Geometry: final body of the model. Coordinates: model frame, mm. Face numbers are marked on the shaded views. A direction names the side the tool comes from. Coordinates: 2 decimals unless noted, no trailing zeros. Order: outer loops, then holes, each group sorted by start corner. A loop starts at its lowest first (then second) coordinate and runs counter-clockwise, first axis right, second up. Notation, with made-up numbers: (28.5, 61.25) -> (60.5, 61.25) arc R27 cw to (60.5, 96.25) -> close; hole circle Ø7 at (8.25, -17.5). An arc over 180 degrees is marked (long way). Use CSV: the item, a comma, the result in double quotes. Start each with the question number.
Autodesk Inventor part; units mm, degrees
ref_plane "Work Plane1" through (0, 41.6, 0) normal (0, 1, 0) x (1, 0, 0)
ref_plane "Work Plane2" through (0, 50.6, 0) normal (0, 1, 0) x (1, 0, 0)
ref_plane "YZ Plane" through (0, 0, 0) normal (1, 0, 0) x (0, 1, 0)
sketch "Sketch1" plane through (0, 0, 0) normal (0, 1, 0) x (-1, 0, 0)
  circle A0 centre (0, 0) radius 13.75
  dimension "d0" = 27.5
extrude "Extrusion1" add sketch "Sketch1" along normal blind 46.6
sketch "Sketch2" plane through (0, 46.6, 0) normal (0, 1, 0) x (1, 0, 0)
  circle A0 centre (0, 0) radius 13.75
  circle A1 centre (0, 0) radius 5
  dimension "d3" = 10
extrude "Extrusion2" add sketch "Sketch2" along normal blind 3 contours A1
sketch "Sketch3" plane through (0, 46.6, 0) normal (0, 1, 0) x (1, 0, 0)
  circle A0 centre (0, 0) radius 5
  circle A1 centre (0, 0) radius 5
  circle A2 centre (0, 0) radius 13.75
  circle A3 centre (0, 0) radius 13.75
  line L0 (-13.75, 0) -> (13.75, 0)
  point P0 (-8, 0)
  point P1 (8, 0)
  dimension "d6" = 16
  dimension "d7" = 5.75
  dimension "d8" = 5.75
hole "Hole1" at (-8, 46.6, 0) at (8, 46.6, 0) direction (0, -1, 0) diameter 2.459 depth 3
ref_plane "Work Plane1" through (0, 41.6, 0) normal (0, 1, 0) x (1, 0, 0)
sketch "Sketch4" plane through (0, 41.6, 0) normal (0, 1, 0) x (1, 0, 0)
  circle A0 centre (0, 0) radius 15
  dimension "d17" = 30
extrude "Extrusion3" add sketch "Sketch4" against normal blind 27.7
sketch "Sketch5" plane through (0, 0, 0) normal (0, -1, 0) x (1, 0, 0)
  circle A0 centre (0, 0) radius 5
  dimension "d20" = 10
extrude "Extrusion4" add sketch "Sketch5" along normal blind 2.7
sketch "Sketch6" plane through (0, 0, 0) normal (0, -1, 0) x (1, 0, 0)
  circle A0 centre (0, 0) radius 5
  circle A1 centre (0, 0) radius 5
  circle A2 centre (0, 0) radius 13.75
  circle A3 centre (0, 0) radius 13.75
  line L0 (13.75, 0) -> (-13.75, 0)
  line L1 (-11.25, 1.35) -> (-11.75, 1.35)
  line L2 (-11.75, 1.35) -> (-11.75, -1.35)
  line L3 (-11.75, -1.35) -> (-11.25, -1.35)
  line L4 (-11.25, -1.35) -> (-11.25, 1.35)
  line L5 (11.25, 1.35) -> (10.75, 1.35)
  line L6 (10.75, 1.35) -> (10.75, -1.35)
  line L7 (10.75, -1.35) -> (11.25, -1.35)
  line L8 (11.25, -1.35) -> (11.25, 1.35)
  dimension "d23" = 22
  dimension "d24" = 0.5
  dimension "d25" = 0.5
  dimension "d26" = 11.25
  dimension "d27" = 11.25
  dimension "d28" = 2.7
  dimension "d29" = 2.7
  dimension "d30" = 1.35
  dimension "d31" = 1.35
extrude "Extrusion5" add sketch "Sketch6" along normal up to surface (2.7 mm away) contours L6 L5 L8 L0 | L0 L8 L7 L6 | L4 L3 L2 L0 | L0 L2 L1 L4
sketch "Sketch7" plane through (0, 49.6, 0) normal (0, 1, 0) x (1, 0, 0)
  circle A0 centre (0, 0) radius 1.15
  dimension "d34" = 2.3
extrude "Extrusion6" add sketch "Sketch7" along normal blind 9.5
ref_plane "Work Plane2" through (0, 50.6, 0) normal (0, 1, 0) x (1, 0, 0)
sketch "Sketch10" plane through (0, 0, 0) normal (1, 0, 0) x (0, 1, 0)
  line L0 (0, -13.75) -> (0, 13.75)
  line L1 (13.9, 13.75) -> (13.9, -13.75)
  line L2 (8.5, 3.8) -> (13.9, 3.8)
  line L3 (13.9, 3.8) -> (13.9, -3.8)
  line L4 (13.9, -3.8) -> (8.5, -3.8)
  line L5 (8.5, -3.8) -> (8.5, 3.8)
  circle A0 centre (11.2, 3.8) radius 2.7
  circle A1 centre (11.2, -3.8) radius 2.7
  line L6 (0, 0) -> (13.9, 0)
  line L7 (13.9, 13.75) -> (13.9, -13.75)
  line L8 (0, -13.75) -> (13.9, -13.75)
  point P0 (11.2, -6.5)
  point P1 (11.2, 6.5)
  dimension "d57" = 8.5
  dimension "d59" = 0
  dimension "d60" = 5.4
  dimension "d61" = 13.9
  dimension "d65" = 3.8
  dimension "d66" = 3.8
  dimension "d80" = 5.4
  dimension "d81" = 5.4
  dimension "d82" = 2.7
  dimension "d83" = 2.7
  dimension "d84" = 13
extrude "Extrusion9" cut sketch "Sketch10" along normal mid plane 31.5 contours L6 L1 A1 L5 | L5 A0 L1 L6 | A1 L4 | L4 A1 | A0 L2 | L2 A0
sketch "Sketch12" plane through (0, 46.6, 0) normal (0, 1, 0) x (1, 0, 0)
  circle A0 centre (0, 0) radius 1.15
  circle A1 centre (0, 0) radius 5
  circle A2 centre (-8, 0) radius 1.2295
  circle A3 centre (8, 0) radius 1.2295
  circle A4 centre (0, 0) radius 5
  circle A5 centre (0, 0) radius 13.75
  circle A6 centre (0, 0) radius 13.75
  line L0 (-13.75, 0) -> (13.75, 0)
  line L1 (0, 13.75) -> (0, -13.75)
  circle A7 centre (0, 0) radius 6.7705
  circle A8 centre (0, 0) radius 9.8705
  line L2 (-2.75, 6.1869) -> (-4.0091, 9.0196)
  line L3 (-6.3854, 2.2508) -> (-9.3091, 3.2814)
  line L4 (2.75, 6.1869) -> (4.0091, 9.0196)
  line L5 (6.3854, 2.2508) -> (9.3091, 3.2814)
  circle A9 centre (-8, 0) radius 1.2295
  circle A10 centre (8, 0) radius 1.2295
  line L6 (-2.75, -6.1869) -> (-4.0091, -9.0196)
  line L7 (-6.3854, -2.2508) -> (-9.3091, -3.2814)
  line L8 (2.75, -6.1869) -> (4.0091, -9.0196)
  line L9 (6.3854, -2.2508) -> (9.3091, -3.2814)
  point P0 (0, 6.7705)
  point P1 (0, 9.8705)
  point P2 (-8, 1.2295)
  point P3 (8, 1.2295)
  dimension "d85" = 3.1
  dimension "d86" = 5.5
  dimension "d87" = 4.0091
  dimension "d88" = 4.0091
  dimension "d89" = 1.5
  dimension "d90" = 1.5
  dimension "d91" = 1.2295
  dimension "d92" = 2.459
  dimension "d93" = 2.459
  dimension "d94" = 1.2295
extrude "Extrusion11" cut sketch "Sketch12" against normal blind 10 contours A7 L4 A8 L5 | L9 A8 L8 A7 | A7 L3 A8 L2 | L6 A8 L7 A7
fillet "Fillet1" radius 1 16 edges at (-4.0091, 41.6, -9.0196) (-2.75, 41.6, -6.1869) (-6.3854, 41.6, -2.2508) (-9.3091, 41.6, -3.2814) (9.3091, 41.6, -3.2814) (6.3854, 41.6, -2.2508) (4.0091, 41.6, -9.0196) (9.3091, 41.6, 3.2814) (6.3854, 41.6, 2.2508) (4.0091, 41.6, 9.0196) (2.75, 41.6, 6.1869) (-4.0091, 41.6, 9.0196) (-9.3091, 41.6, 3.2814) (-6.3854, 41.6, 2.2508) (-2.75, 41.6, 6.1869) (2.75, 41.6, -6.1869)
sketch "Sketch13" plane through (0, -2.7, 0) normal (0, -1, 0) x (1, 0, 0)
  circle A0 centre (0, 0) radius 3.25
  dimension "d98" = 6.5
extrude "Extrusion12" add sketch "Sketch13" along normal blind 1
sketch "Sketch14" plane through (0, -3.7, 0) normal (0, -1, 0) x (1, 0, 0)
  circle A0 centre (0, 0) radius 1.2
  dimension "d101" = 2.4
extrude "Extrusion13" add sketch "Sketch14" along normal blind 1.1
equation "\"d26\" = d27"
equation "\"d30\" = d31"
equation "\"d65\" = d66"
equation "\"d82\" = 0.5 * d80"
equation "\"d83\" = 0.5 * d81"
equation "\"d87\" = d88"
equation "\"d41\" = d42"
properties part number "rs390" material "Steel, Mild"
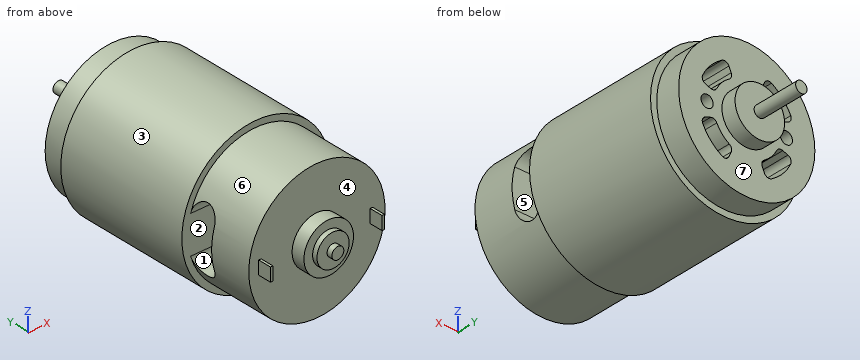
(1) Access query for the marked faces 5, 6 and 7. Directions: +Z, -Z, +X, -X, +Y, -Y. A direction counts if a zero-diameter tool reaches every point of the face in a straight line with its end or side. Return the directions, or none.
(2) Mould query, pull axis Y, two halves, no side actions, for the marked faces 1, 2, 3 and 4. Classes: pulls with the +Y half, pulls with the -Y half, needs draft (parallel to the pull), parting line crosses it, or undercut.
(3) Line query: line 1 (X direction, y = 45.45, z = 0); line 2 (Y direction, x = -1.5, z = -2); line 3 (Z direction, x = 8, y = 44.95). Output: solid intervals per line, ascending. Write a range as from..to.
(4) Section B-B (y = 11.2). Return loops of the section in (x, z).
(5) Section A-A (z = -11). Return loops of the section in (x, y).
(6) First-contact query: pin 1 (4.5 mm diameter, centred on x = -6.5, z = 5.5, fed in from +Y); pin 2 (0.8 mm diameter, centred on y = -2, z = -0.5, fed in from +X); pin 3 (6 mm diameter, centred on x = 4.5, z = 2, fed in from -Y). Flat tips, straight axial feed; report the tip coordinate or a pass-through.
(7) Section C-C (y = 1.5). Return loops of the section in (x, z).
(8) Section D-D (y = 22.5). Return loops of the section in (x, z).
Check sheet entries:
1,face 5,"+X, -X"
1,face 6,"-Y"
1,face 7,"+Y"
2,face 1,"undercut"
2,face 2,"undercut"
2,face 3,"needs draft"
2,face 4,"pulls with the -Y half"
3,line 1,"x = -13.75..-9.23, -6.77..6.77, 9.23..13.75"
3,line 2,"y = -3.7..8.5, 13.9..49.6"
3,line 3,"z = -11.18..-5.78, -2.82..-1.23, 1.23..2.82, 5.78..11.18"
4,outline,"(-12.12, -6.5) arc R13.75 ccw to (12.12, -6.5) -> close; (-12.12, 6.5) -> (12.12, 6.5) arc R13.75 ccw to start"
5,outline,"(-10.2, 13.9) -> (-8.25, 13.9) -> (-8.25, 0) -> (8.25, 0) -> (8.25, 13.9) -> (10.2, 13.9) -> (10.2, 41.6) -> (8.25, 41.6) -> (8.25, 46.6) -> (-8.25, 46.6) -> (-8.25, 41.6) -> (-10.2, 41.6) -> close"
6,pin 1,"stops at y = 46.6"
6,pin 2,"stops at x = 11.25"
6,pin 3,"stops at y = -3.7"
7,outline,"circle Ø27.5 at (0, 0)"
8,outline,"circle Ø30 at (0, 0)"
